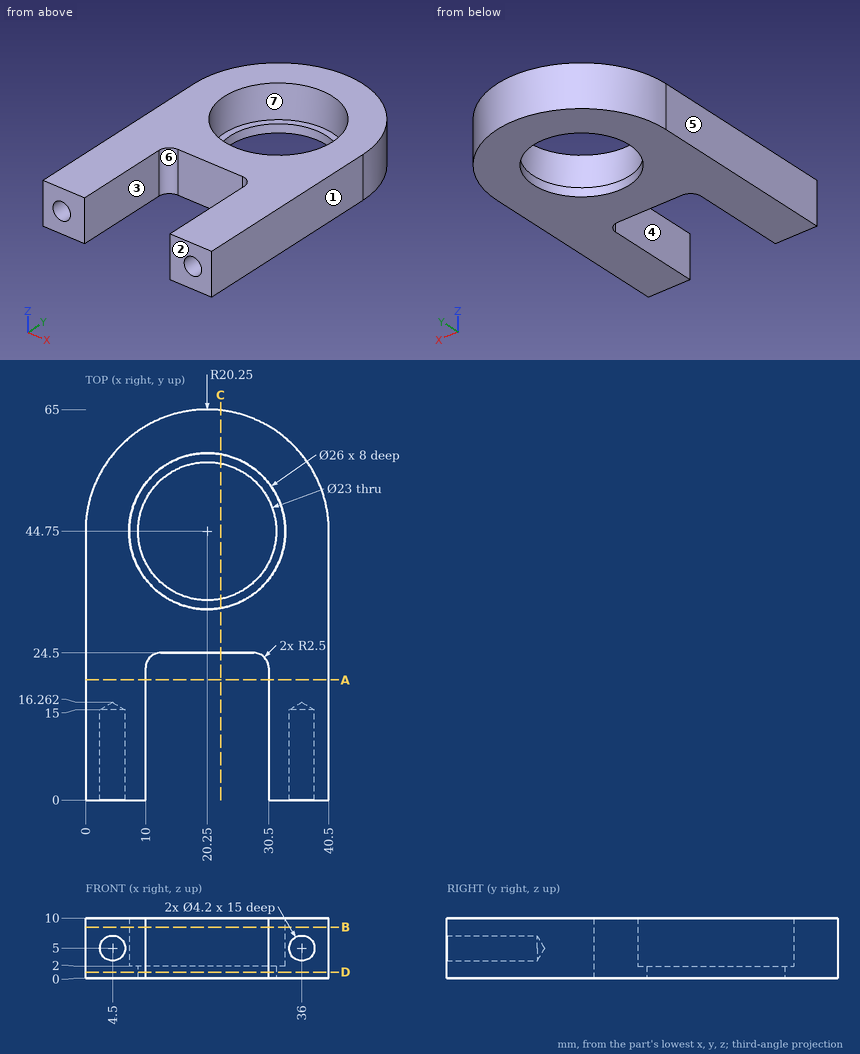
Check sheet for the drawn part. Datum: minimum x, y, z corner. Units: mm. A direction names the side the tool comes from. Coordinates: 2 decimals unless noted, no trailing zeros. Order: outer loops, then holes, each group sorted by start corner. A loop starts at its lowest first (then second) coordinate and runs counter-clockwise, first axis right, second up. Notation, with made-up numbers: (61, 81) - (100, 81) arc R17 ccw to (100, 112) - close; hole circle Ø7 at (36.25, 27). An arc over 180 degrees is marked (long way). Return JSON: item names as keys, results as strings.
(1) Section check A-A, the plane y = 20. Record the cut outline in (x, z).
Filled sheet:
{"outline": "(0, 0) - (10, 0) - (10, 10) - (0, 10) - close; (30.5, 0) - (40.5, 0) - (40.5, 10) - (30.5, 10) - close"}
(2) Section check D-D, the plane z = 1. Record the cut outline in (x, y), and give its area (3 significant figures).
Filled sheet:
{"outline": "(0, 0) - (10, 0) - (10, 22) arc R2.5 cw to (12.5, 24.5) - (28, 24.5) arc R2.5 cw to (30.5, 22) - (30.5, 0) - (40.5, 0) - (40.5, 44.75) arc R20.25 ccw to (0, 44.75) - close; hole circle Ø23 at (20.25, 44.75)", "area": "1,540 mm^2"}
(3) Thickness scan on line 1 along Y through (x, z) = (20.25, 8); line 2 along X through (y, z) = (21, 5.5); line 3 along Y through (x, z) = (20.25, 1.4). Record the ranges inside material, lowest first.
Filled sheet:
{"line 1": "y = 24.5 to 31.75, 57.75 to 65", "line 2": "x = 0 to 10, 30.5 to 40.5", "line 3": "y = 24.5 to 33.25, 56.25 to 65"}
(4) Section check C-C, the plane x = 22.5. Record the cut outline in (y, z) (1 decimal).
Filled sheet:
{"outline": "(24.5, 0) - (33.5, 0) - (33.5, 2) - (31.9, 2) - (31.9, 10) - (24.5, 10) - close; (56, 0) - (64.9, 0) - (64.9, 10) - (57.6, 10) - (57.6, 2) - (56, 2) - close"}
(5) Section check B-B, the plane z = 8.5. Record the cut outline in (x, y), and give its area (3 significant figures).
Filled sheet:
{"outline": "(0, 0) - (10, 0) - (10, 22) arc R2.5 cw to (12.5, 24.5) - (28, 24.5) arc R2.5 cw to (30.5, 22) - (30.5, 0) - (40.5, 0) - (40.5, 44.75) arc R20.25 ccw to (0, 44.75) - close; hole circle Ø26 at (20.25, 44.75)", "area": "1,430 mm^2"}
(6) Access from +Z, -Z, +X, -X, +Y, -Y to the whole of each face (thin tool, end or side, straight path). Record for the marked faces 5, 6 and 7.
Filled sheet:
{"face 5": "+Z, -Z, -X, +Y, -Y", "face 6": "+Z, -Z, -Y", "face 7": "+Z"}
(7) Go/stop test with flat-tipped pins: pin 1 (4 mm diameter, centred on x = 4.5, z = 5, fed in from -Y); pin 2 (4 mm diameter, centred on x = 12.5, y = 53.5, fed in from -Z); pin 3 (3 mm diameter, centred on x = 19, z = 4, fed in from -Y); pin 4 (4 mm diameter, centred on x = 26, z = 5.5, fed in from +Y). Record where each tip stops, or that it passes through.
Filled sheet:
{"pin 1": "stops at y = 15.06", "pin 2": "stops at z = 0", "pin 3": "stops at y = 24.5", "pin 4": "stops at y = 64.65"}
(8) Mould release check, pull along X, two halves, no side actions. Record for the marked faces 1, 2, 3 and 4: pulls with the +X half, pulls with the -X half, needs draft (parallel to the pull), parting line crosses it, or undercut.
Filled sheet:
{"face 1": "pulls with the +X half", "face 2": "needs draft", "face 3": "undercut", "face 4": "undercut"}
